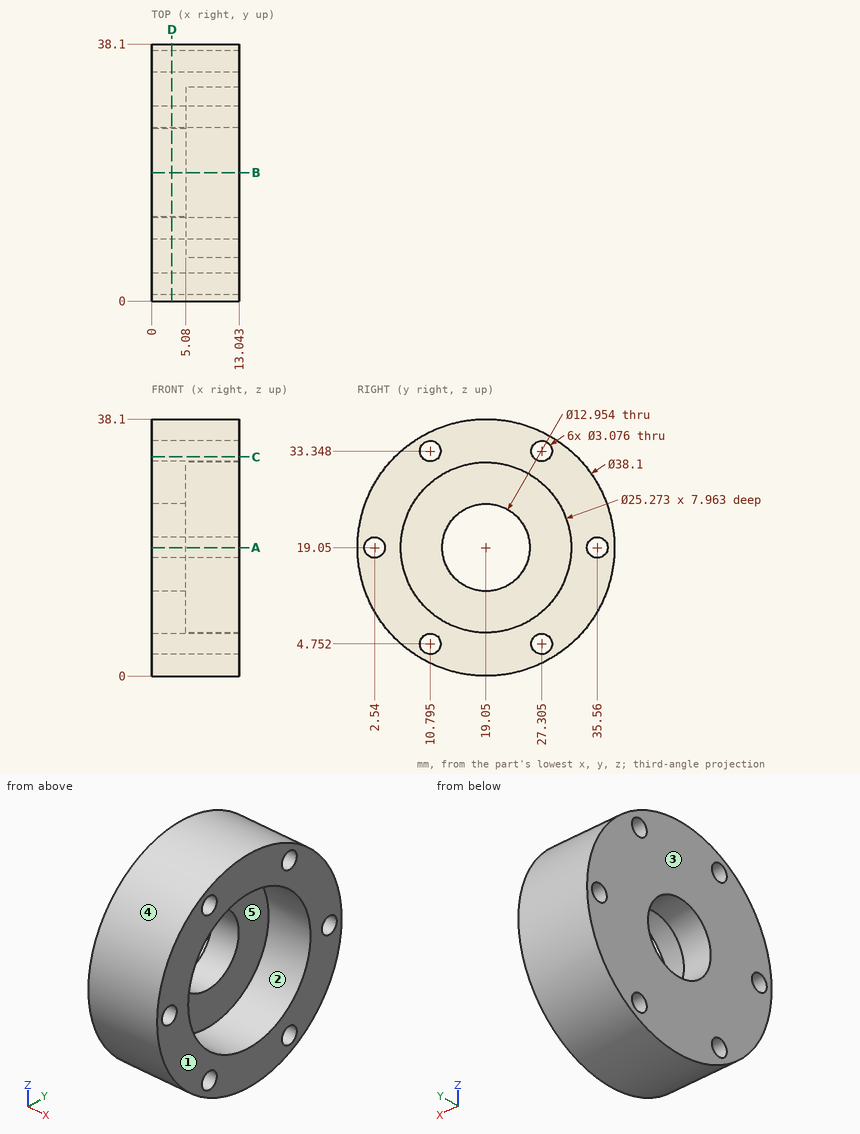
Here's the drawing with two shaded views (mm, measured from the low corner). I have some questions. A direction names the side the tool comes from. Give positions to 0.01 mm unless a question says otherwise; leave off trailing zeros. Order: outer loops, then holes, each group sorted by start corner. A loop starts at its lowest first (then second) coordinate and runs counter-clockwise, first axis right, second up. Notation, with made-up numbers: (24.25, 50) -> (48.25, 50) arc R16 ccw to (48.25, 70) -> close; hole circle Ø1 at (66.25, -30.75). An arc over 180 degrees is marked (long way). One line per item, written item: value. Start each with the question number.
1. Will these pins go through, and if not, where does the flat tip stop? pin 1 Ø1.8 at (y, z) = (10.8, 4.75) entering from -X; pin 2 Ø6 at (x, z) = (11.5, 7) entering from +Y; pin 3 Ø20.5 at (y, z) = (19.05, 19.05) entering from +X; pin 4 Ø4 at (x, z) = (2.5, 27) entering from -Y.
2. For the marked faces 1 and 2, which set-ups out of +Z, -Z, +X, -X, +Y, -Y let a thin tool reach every point of the face, with its end or its side?
3. I need wall thicknesses on probe 1 along Y at (x, z) = (10.25, 19); probe 2 along Z at (x, y) = (1.15, 19.05); probe 3 along Z at (x, y) = (6, 27) (1 decimal). Which ranges of each line are inside material? Lowest first, please. Write a range as from..to.
4. Imagine slicing it at B-B, the plane y = 19.05. List the corners of the cut face in (x, z) for me.
5. Imagine slicing it at A-A, the plane z = 19.05. List the corners of the cut face in (x, y) for me, plus the area to 3 significant figures.
6. Imagine slicing it at D-D, the plane x = 3. Count the separate pieces of the cut face and the enclosed holes in it, plus the area to 3 significant figures.
7. We'd pull the mould along Y, two halves only. Please class the marked faces 3, 4 and 5: released by +Y, released by -Y, zero draft, split by the parting line, or undercut.
8. Imagine slicing it at C-C, the plane z = 32.5. List the corners of the cut face in (x, y) for me.
Values follow:
1. pin 1: passes through
1. pin 2: stops at y = 35.81
1. pin 3: stops at x = 5.08
1. pin 4: stops at y = 0.95
2. face 1: +Z, -Z, +X, +Y, -Y
2. face 2: +X
3. probe 1: y = 0..1, 4.08..6.41, 31.69..34.02, 37.1..38.1
3. probe 2: z = 0..12.57, 25.53..38.1
3. probe 3: z = 1.7..3.2, 6.3..9.2, 28.9..31.8, 34.9..36.4
4. outline: (0, 0) -> (13.04, 0) -> (13.04, 6.41) -> (5.08, 6.41) -> (5.08, 12.57) -> (0, 12.57) -> close; (0, 25.53) -> (5.08, 25.53) -> (5.08, 31.69) -> (13.04, 31.69) -> (13.04, 38.1) -> (0, 38.1) -> close
5. outline: (0, 0) -> (13.04, 0) -> (13.04, 1) -> (0, 1) -> close; (0, 4.08) -> (13.04, 4.08) -> (13.04, 6.41) -> (5.08, 6.41) -> (5.08, 12.57) -> (0, 12.57) -> close; (0, 25.53) -> (5.08, 25.53) -> (5.08, 31.69) -> (13.04, 31.69) -> (13.04, 34.02) -> (0, 34.02) -> close; (0, 37.1) -> (13.04, 37.1) -> (13.04, 38.1) -> (0, 38.1) -> close
5. area: 150 mm2
6. separate pieces: 1
6. enclosed holes: 7
6. area: 964 mm2
7. face 3: zero draft
7. face 4: split by the parting line
7. face 5: undercut
8. outline: (0, 5.56) -> (13.04, 5.56) -> (13.04, 9.51) -> (0, 9.51) -> close; (0, 12.08) -> (13.04, 12.08) -> (13.04, 26.02) -> (0, 26.02) -> close; (0, 28.59) -> (13.04, 28.59) -> (13.04, 32.54) -> (0, 32.54) -> close
